Here's how the part is built. I have some questions about the finished solid (model axes, mm). A direction names the side the tool comes from. Round coordinates to 2 decimals unless told otherwise and drop trailing zeros. Order: outer loops, then holes, each group sorted by start corner. A loop starts at its lowest first (then second) coordinate and runs counter-clockwise, first axis right, second up.
```python
from build123d import *

# Parameters (mm, degrees)
F1_DEPTH = 28.575
F2_R     = 12.7
F3_DEPTH = 9.525
F4_R     = 2.54


# Not quite as in the source:
# - a pattern or mirror of a feature is missing from the dataset's text; its kind, count and spacing are read off the source's solid


with BuildPart() as f1:
    # F0 (on Front) → F1 (new body, symmetric)
    with BuildSketch(Plane.XZ):
        with BuildLine():
            Line((-152.4, 0), (0, 0))
            Line((0, 0), (0, 12.7))
            Line((0, 12.7), (-105.7247139353, 37.1224254179))
            ThreePointArc((-105.7247139353, 37.1224254179), (-138.0159397973, 29.8188564424), (-152.4, 0))
        make_face()
    extrude(amount=F1_DEPTH, both=True)

    # F2 (on face) → F3 (cut)
    with BuildSketch(Plane.XZ.offset(28.575)):
        with Locations((-127, 10.16)):
            Circle(F2_R)
        with Locations((-31.75, 7.62)):
            Circle(F2_R)
    f3 = extrude(amount=-F3_DEPTH, mode=Mode.SUBTRACT)

    # F3_copies: F3 across plane
    add(f3.mirror(Plane.ZX), mode=Mode.SUBTRACT)

    # F4
    f4_edges = [f1.edges().sort_by_distance(p)[0] for p in [
        (-25.256061, -23.8125, 18.534154),
        (-32.799092, -23.8125, 20.276595),
        (-41.91, -23.8125, 0),
        (-21.59, -23.8125, 0),
        (-134.62, -23.8125, 0),
        (-119.38, -23.8125, 0),
        (-21.59, 23.8125, 0),
        (-41.91, 23.8125, 0),
        (-119.38, 23.8125, 0),
        (-134.62, 23.8125, 0),
        (-32.799092, 23.8125, 20.276595),
        (-25.256061, 23.8125, 18.534154),
    ]]
    fillet(f4_edges, radius=F4_R)


solid = f1.part
```
1) If we section it at A-A (y = 24.5): Write out the boundary of the cut face in (x, z).
2) If we section it at D-D (y = 15): Write out the boundary of the cut face in (x, z), plus the area to 3 significant figures.
3) For faces 5 (the flat face through (-96, -28.575, 15)), 6 (the cylindrical face through (-19.066, 23.879, 8.253)), 7 (the cylindrical face through (-44.1, -23.9, 1)), which set-ups out of +Z, -Z, +X, -X, +Y, -Y let a thin tool reach every point of the face, with its end or its side?
4) We'd pull the mould along X, two halves only. Please class faces 1 (the flat face through (-10, -28.575, 9)), 2 (the cylindrical face through (-38.7, 23.9, 20.2)), 3 (the cylindrical face through (-126.628, 23.879, 22.855)), 4 (the cylindrical face through (-19.992, 23.879, 15.874)): +X half, -X half, draft (parallel to the pull), parting line (faces both ways), or undercut.
5) I'm going to push flat-ended pins straight in: pin 1 (17.5 mm diameter, centred on x = -31.5, z = 8, fed in from +Y); pin 2 (4 mm diameter, centred on x = -84.5, y = -19, fed in from +Z); pin 3 (8 mm diameter, centred on y = 0, z = 30.5, fed in from -X). Where does each tip first touch, or does it pass through?
6) I need wall thicknesses on line 1 (X direction, y = 23.5, z = 3.5); line 2 (X direction, y = -26.5, z = 10.16); line 3 (Y direction, x = -127.5, z = 20). Which ranges of each line are inside material? Lowest first, please.
7) If we section it at B-B (x = -127): Write out the boundary of the cut face in (y, z) (3 decimals), plus the area to 3 significant figures.
8) If we section it at C-C (z = 10.16): Write out the boundary of the cut face in (x, y) (3 decimals), plus the area to 3 significant figures.
Solutions:
1. outline: (-152.4, 0) - (-140.2, 0) arc R2.54 ccw to (-138, 3.81) arc R12.7 cw (long way) to (-116, 3.81) arc R2.54 ccw to (-113.8, 0) - (-46.12, 0) arc R2.54 ccw to (-43.72, 3.39) arc R12.7 cw to (-39.6, 17.61) arc R2.54 ccw to (-40.6, 22.08) - (-105.72, 37.12) arc R38.1 ccw to start; (-20.32, 13.15) arc R12.7 cw to (-19.78, 3.39) arc R2.54 ccw to (-17.38, 0) - (0, 0) - (0, 12.7) - (-17.46, 16.73) arc R2.54 ccw to start
2. outline: (-152.4, 0) - (0, 0) - (0, 12.7) - (-105.72, 37.12) arc R38.1 ccw to start
2. area: 4,100 mm2
3. face 5: +Z, -Z, +X, -X, -Y
3. face 6: +Y
3. face 7: -Y
4. face 1: draft
4. face 2: +X half
4. face 3: undercut
4. face 4: undercut
5. pin 1: stops at y = 19.05
5. pin 2: stops at z = 32.68
5. pin 3: stops at x = -141.67
6. line 1: x = -152.24 to -137.85, -116.15 to -43.76, -19.74 to 0
6. line 2: x = -151.02 to -139.7, -114.3 to -44.19, -19.31 to 0
6. line 3: y = -19.05 to 19.05
7. outline: (-28.575, 22.86) - (-19.05, 22.86) - (-19.05, 0) - (19.05, 0) - (19.05, 22.86) - (28.575, 22.86) - (28.575, 35.921) - (-28.575, 35.921) - close
7. area: 1,620 mm2
8. outline: (-151.02, -28.575) - (-139.7, -28.575) - (-139.7, -19.05) - (-114.3, -19.05) - (-114.3, -28.575) - (-44.193, -28.575) - (-44.193, -19.05) - (-19.307, -19.05) - (-19.307, -28.575) - (0, -28.575) - (0, 28.575) - (-19.307, 28.575) - (-19.307, 19.05) - (-44.193, 19.05) - (-44.193, 28.575) - (-114.3, 28.575) - (-114.3, 19.05) - (-139.7, 19.05) - (-139.7, 28.575) - (-151.02, 28.575) - close
8. area: 7,670 mm2
